Check sheet for the drawn part. Datum: minimum x, y, z corner. Units: mm. A direction names the side the tool comes from. Give positions to 0.01 mm unless a question says otherwise; leave off trailing zeros. Write each loop counter-clockwise with the first axis right and the second up, starting at its lowest first coordinate (ties: lowest second). Pieces come first, ordered by that corner, then holes. Notation, with made-up numbers: (-4, 6.25) - (2, 6.25) arc R30 ccw to (2, 28.25) - close; hole circle Ø10 at (18, 45.5). An arc over 180 degrees is marked (long way). One line per question, with ' | ' between items. Start each with the question number.
Q1. Release check for a two-part mould opening along Y. For the marked faces 3, 4 and 5 record: +Y half, -Y half, draft (parallel to the pull), parting line (faces both ways), or undercut.
Q2. Gauge pin test, flat ends, axial feed: P1, Ø0.8, axis at y = 6.5, z = 1, coming from the +X side (1 decimal); P2, Ø0.8, axis at x = 21, z = 0.5, coming from the -Y side (1 decimal); P3, Ø4, axis at x = 6.35, y = 6.35, coming from the +Z side. Record the tip position at first contact, or that the pin passes through.
Q3. Section check A-A on x = 18.75. Record the boundary of the cut face in (y, z).
Q4. Set-up check for the marked faces 1 and 2: record each of +Z, -Z, +X, -X, +Y, -Y from which the full face is reachable in a straight line by a thin tool's end or side.
Q5. Section check B-B on y = 6. Record the boundary of the cut face in (x, z) (1 decimal).
Q6. Thickness scan on L1, parallel to Y at x = 6.35, z = 0.95 (1 decimal); L2, parallel to X at y = 5.5, z = 1.1 (1 decimal); L3, parallel to Y at x = 21.75, z = 0.65 (1 decimal). Record the ranges inside material, lowest first. Write a range as [from, to].
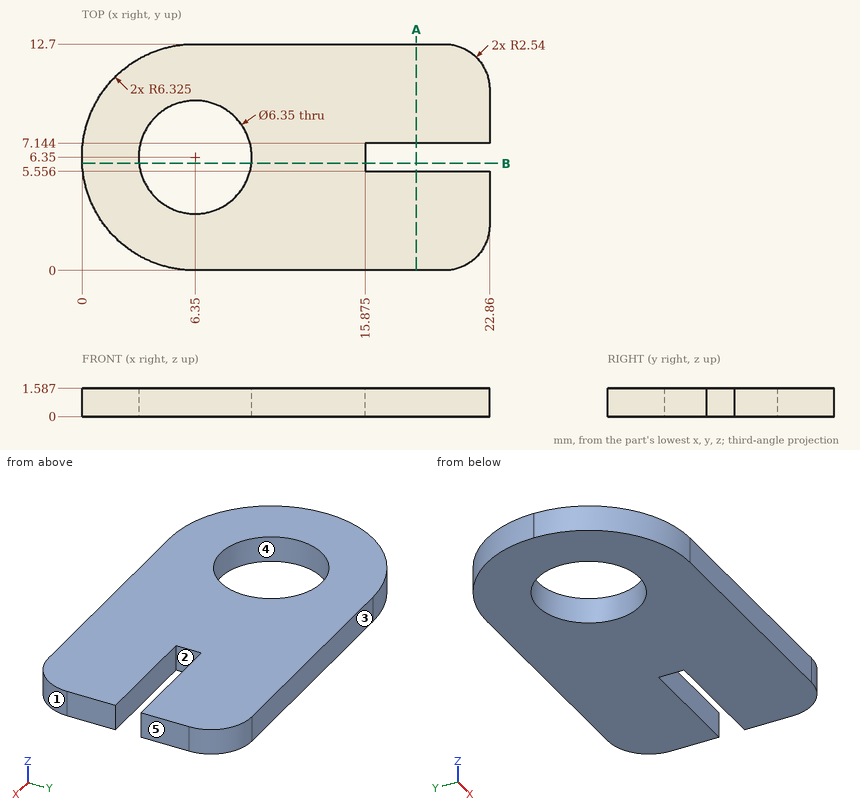
Working result:
1) face 3: +Y half | face 4: undercut | face 5: draft
2) P1: stops at x = 15.9 | P2: stops at y = 0 | P3: passes through
3) outline: (0, 0) - (5.56, 0) - (5.56, 1.59) - (0, 1.59) - close; (7.14, 0) - (12.7, 0) - (12.7, 1.59) - (7.14, 1.59) - close
4) face 1: +Z, -Z, +X, -Y | face 2: +Z, -Z, +X
5) outline: (0, 0) - (3.2, 0) - (3.2, 1.6) - (0, 1.6) - close; (9.5, 0) - (15.9, 0) - (15.9, 1.6) - (9.5, 1.6) - close
6) L1: y = [0, 3.2], [9.5, 12.7] | L2: x = [0.1, 3.3], [9.4, 22.9] | L3: y = [0.4, 5.6], [7.1, 12.3]
